The listing builds one solid part. Answer for the finished solid, in the listing's coordinates (mm). A direction names the side the tool comes from. Coordinates: 2 decimals unless noted, no trailing zeros. Order: outer loops, then holes, each group sorted by start corner. A loop starts at its lowest first (then second) coordinate and runs counter-clockwise, first axis right, second up. Notation, with made-up numbers: (72.25, 76) - (102.25, 76) arc R36 cw to (102.25, 110) - close; hole circle Ø4 at (0, 6.5). An arc over 180 degrees is marked (long way). One line per item, written item: value. Start each with the question number.
```python
from build123d import *

# Parameters (mm, degrees)
SKETCH1_W           = 25.4
SKETCH1_H           = 12.7
BOSS_EXTRUDE1_DEPTH = 2.54
BOSS_EXTRUDE2_DEPTH = 5.08
SKETCH3_R           = 3.175
CUT_EXTRUDE1_DEPTH  = 26.4


with BuildPart() as part:
    # Sketch1 → Boss-Extrude1 (new body)
    with BuildSketch(Plane(origin=(0, 0, 0), x_dir=(1, 0, 0), z_dir=(0, 1, 0))):
        Rectangle(SKETCH1_W, SKETCH1_H)
    extrude(amount=BOSS_EXTRUDE1_DEPTH)

    # Sketch2 → Boss-Extrude2 (add)
    with BuildSketch(Plane(origin=(12.7, 0, 0), x_dir=(0, 0, -1), z_dir=(1, 0, 0))):
        with BuildLine():
            Line((-6.35, 2.54), (-3.062998127, 14.807257994))
            ThreePointArc((-3.062998127, 14.807257994), (0, 16.07599336), (3.062998127, 14.807257994))
            Line((3.062998127, 14.807257994), (6.35, 2.54))
            Line((6.35, 2.54), (-6.35, 2.54))
        make_face()
    boss_extrude2 = extrude(amount=-BOSS_EXTRUDE2_DEPTH)

    # Mirror1: Boss-Extrude2 across plane
    add(boss_extrude2.mirror(Plane(origin=(0, 0, 0), x_dir=(0, 0, 1), z_dir=(1, 0, 0))))

    # Sketch3 → Cut-Extrude1 (cut, through all)
    with BuildSketch(Plane(origin=(12.7, 0, 0), x_dir=(0, 0, -1), z_dir=(1, 0, 0))):
        with Locations((0, 10.16)):
            Circle(SKETCH3_R)
    extrude(amount=-CUT_EXTRUDE1_DEPTH, mode=Mode.SUBTRACT)


solid = part.part
```
(1) Consider probe 1 along X at (y, z) = (4.5, 0.5); probe 2 along Y at (x, z) = (9.5, 0) (3 decimals); probe 3 along Y at (x, z) = (-4.25, 2). Determine where each line is inside the solid, lowest interval first.
(2) The part is cut by section B-B on z = 0. Determine the outline of the cut face in (x, y) (3 decimals).
(3) For faces 4 (the face through (7.62, 6, 0)), 5 (the face through (10.2, 8.59, 4.73)), determine the directions among +Z, -Z, +X, -X, +Y, -Y from which every point of the face is accessible in a straight line to the end or side of a thin tool.
(4) The part is cut by section C-C on y = 12.75. Determine the outline of the cut face in (x, z), plus the area to 3 significant figures.
(5) Flat-ended cylindrical pins translate along their axes: pin 1 Ø6.5 at (y, z) = (11.5, 2) entering from -X; pin 2 Ø5 at (y, z) = (10.16, 0) entering from -X; pin 3 Ø8 at (x, y) = (-7, 12) entering from +Z; pin 4 Ø4 at (x, z) = (2, -1) entering from +Y. Find the tip coordinate at first contact, or state that the pin passes through.
(6) The part is cut by section D-D on x = 10.5. Determine the outline of the cut face in (y, z) (3 decimals), plus the area to 3 significant figures.
(7) For a pull along Y with two mould halves and no side action, classify faces 1 (the face through (-7.62, 6, 0)), 2 (the face through (10.2, 13.31, 0.41)), 3 (the face through (0, 2.54, 0)) as pulls with the +Y half, pulls with the -Y half, needs draft (parallel to the pull), parting line crosses it, or undercut.
(8) The part is cut by section A-A on y = 4.5. Determine the outline of the cut face in (x, z).
Completed:
1. probe 1: x = -12.7 to -7.62, 7.62 to 12.7
1. probe 2: y = 0 to 6.985, 13.335 to 16.076
1. probe 3: y = 0 to 2.54
2. outline: (-12.7, 0) - (12.7, 0) - (12.7, 6.985) - (7.62, 6.985) - (7.62, 2.54) - (-7.62, 2.54) - (-7.62, 6.985) - (-12.7, 6.985) - close; (-12.7, 13.335) - (-7.62, 13.335) - (-7.62, 16.076) - (-12.7, 16.076) - close; (7.62, 13.335) - (12.7, 13.335) - (12.7, 16.076) - (7.62, 16.076) - close
3. face 4: +Z, -Z, +Y
3. face 5: +Z, +X, -X, +Y
4. outline: (-12.7, -3.61) - (-7.62, -3.61) - (-7.62, -1.84) - (-12.7, -1.84) - close; (-12.7, 1.84) - (-7.62, 1.84) - (-7.62, 3.61) - (-12.7, 3.61) - close; (7.62, -3.61) - (12.7, -3.61) - (12.7, -1.84) - (7.62, -1.84) - close; (7.62, 1.84) - (12.7, 1.84) - (12.7, 3.61) - (7.62, 3.61) - close
4. area: 36.1 mm2
5. pin 1: stops at x = -12.7
5. pin 2: passes through
5. pin 3: stops at z = 4.87
5. pin 4: stops at y = 2.54
6. outline: (0, -6.35) - (2.54, -6.35) - (14.807, -3.063) arc R4.332 ccw to (14.807, 3.063) - (2.54, 6.35) - (0, 6.35) - close; hole circle Ø6.35 at (10.16, 0)
6. area: 121 mm2
7. face 1: needs draft
7. face 2: undercut
7. face 3: pulls with the +Y half
8. outline: (-12.7, -5.82) - (-7.62, -5.82) - (-7.62, 5.82) - (-12.7, 5.82) - close; (7.62, -5.82) - (12.7, -5.82) - (12.7, 5.82) - (7.62, 5.82) - close
